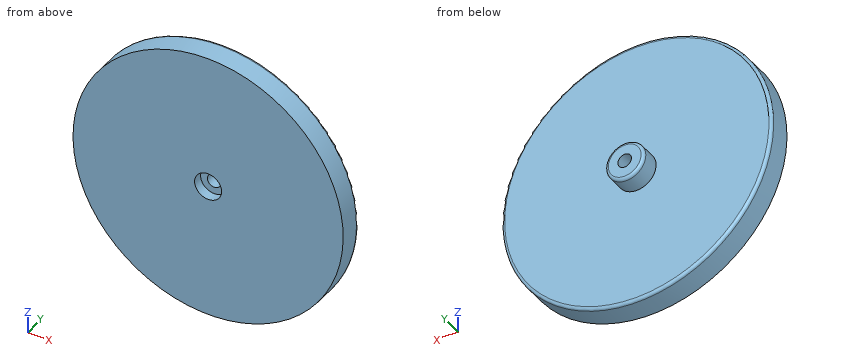
```python
from build123d import *

# Parameters (mm, degrees)
SKETCH1_R           = 35.56
BOSS_EXTRUDE1_DEPTH = 6.35
SKETCH2_R           = 5.08
BOSS_EXTRUDE2_DEPTH = 5.08
SKETCH3_R           = 1.778
CUT_EXTRUDE1_DEPTH  = 12.43
SKETCH4_R           = 3.556
CUT_EXTRUDE2_DEPTH  = 2.54
FILLET1_R           = 0.762
FILLET2_R           = 0.762


with BuildPart() as part:
    # Sketch1 → Boss-Extrude1 (new body)
    with BuildSketch(Plane(origin=(0, 0, 0), x_dir=(1, 0, 0), z_dir=(0, 1, 0))):
        with Locations(Location((0, 0, 0), (0, 0, 270))):  # turned: the seam where the file's is
            Circle(SKETCH1_R)
    extrude(amount=BOSS_EXTRUDE1_DEPTH)

    # Sketch2 → Boss-Extrude2 (add)
    with BuildSketch(Plane(origin=(0, 6.35, 0), x_dir=(1, 0, 0), z_dir=(0, 1, 0))):
        with Locations(Location((0, 0, 0), (0, 0, 270))):  # turned: the seam where the file's is
            Circle(SKETCH2_R)
    extrude(amount=BOSS_EXTRUDE2_DEPTH)

    # Sketch3 → Cut-Extrude1 (cut, through all)
    with BuildSketch(Plane(origin=(0, 11.43, 0), x_dir=(1, 0, 0), z_dir=(0, 1, 0))):
        with Locations(Location((0, 0, 0), (0, 0, 270))):  # turned: the seam where the file's is
            Circle(SKETCH3_R)
    extrude(amount=-CUT_EXTRUDE1_DEPTH, mode=Mode.SUBTRACT)

    # Sketch4 → Cut-Extrude2 (cut)
    with BuildSketch(Plane.XZ):
        with Locations(Location((0, 0, 0), (0, 0, 270))):  # turned: the seam where the file's is
            Circle(SKETCH4_R)
    extrude(amount=-CUT_EXTRUDE2_DEPTH, mode=Mode.SUBTRACT)

    # Fillet1
    fillet1_edges = [part.edges().sort_by_distance(p)[0] for p in [
        (0, 11.43, -5.08),
    ]]
    fillet(fillet1_edges, radius=FILLET1_R)

    # Fillet2
    fillet2_edges = [part.edges().sort_by_distance(p)[0] for p in [
        (0, 6.35, -35.56),
    ]]
    fillet(fillet2_edges, radius=FILLET2_R)


solid = part.part
```
CAD build for the part. Positions are in the model's coordinates, mm. Round coordinates to 2 decimals unless told otherwise and drop trailing zeros. Loops run counter-clockwise (first coordinate to the right, second up) from the corner with the lowest first, then second, coordinate; pieces in that order, holes last. Notation, with made-up numbers: M 48.25,25 L 54.25,25 A3 cw 54.25,29 Z; hole C 1.5,50.25 d1. An arc over 180 degrees is marked long. Return JSON: item names as keys, results as strings. Group by question number.
(1) Wall check: probe 1 along X at (y, z) = (1.35, 0); probe 2 along Y at (x, z) = (-17, -23); probe 3 along X at (y, z) = (5.5, -1). Give the ranges that are in metal, low to high. Write a range as [from, to].
(2) Saw through at A-A, the plane x = 0. List the corners of the cut face in (y, z).
(3) Saw through at C-C, the plane y = 8.25. List the corners of the cut face in (x, z).
(4) Saw through at B-B, the plane z = 0. List the corners of the cut face in (x, y), and give its area (3 significant figures).
(5) Drop flat-ended pins along their axis: P1, Ø4, axis at y = 3.5, z = -10, coming from the -X side; P2, Ø4, axis at x = -28, y = 9, coming from the +Z side; P3, Ø5, axis at x = 12, z = 1, coming from the +Y side; P4, Ø1.5, axis at x = 25, y = 4, coming from the +Z side. Give the stop position or say it passes through.
Answer list:
{
 "1": {"probe 1": "[-35.56, -3.56], [3.56, 35.56]", "probe 2": "[0, 6.35]", "probe 3": "[-35.55, -1.47], [1.47, 35.55]"},
 "2": {"outline": "M 0,-35.56 L 5.59,-35.56 A0.76 ccw 6.35,-34.8 L 6.35,-5.08 L 10.67,-5.08 A0.76 ccw 11.43,-4.32 L 11.43,-1.78 L 2.54,-1.78 L 2.54,-3.56 L 0,-3.56 Z; M 0,3.56 L 2.54,3.56 L 2.54,1.78 L 11.43,1.78 L 11.43,4.32 A0.76 ccw 10.67,5.08 L 6.35,5.08 L 6.35,34.8 A0.76 ccw 5.59,35.56 L 0,35.56 Z"},
 "3": {"outline": "C 0,0 d10.16; hole C 0,0 d3.56"},
 "4": {"outline": "M -35.56,0 L -3.56,0 L -3.56,2.54 L -1.78,2.54 L -1.78,11.43 L -4.32,11.43 A0.76 ccw -5.08,10.67 L -5.08,6.35 L -34.8,6.35 A0.76 ccw -35.56,5.59 Z; M 1.78,2.54 L 3.56,2.54 L 3.56,0 L 35.56,0 L 35.56,5.59 A0.76 ccw 34.8,6.35 L 5.08,6.35 L 5.08,10.67 A0.76 ccw 4.32,11.43 L 1.78,11.43 Z", "area": "453 mm2"},
 "5": {"P1": "x = -34.65", "P2": "through", "P3": "y = 6.35", "P4": "z = 26.01"}
}
